Autodesk Inventor part; units mm, degrees
ref_plane "YZ Plane" through (0, 0, 0) normal (1, 0, 0) x (0, 1, 0)
ref_plane "XZ Plane" through (0, 0, 0) normal (0, 1, 0) x (-1, 0, 0)
ref_plane "XY Plane" through (0, 0, 0) normal (0, 0, 1) x (1, 0, 0)
sketch "Эскиз1" plane through (0, 0, 0) normal (1, 0, 0) x (0, 1, 0)
  line L0 (0.4, 16.4596) -> (0.4, 13.8596)
  line L1 (0.4, 13.8596) -> (2, 13.8596)
  line L2 (2, 13.8596) -> (2, 13.0596)
  line L3 (2, 13.0596) -> (5, 13.0596)
  line L4 (5, 13.0596) -> (5, 1)
  line L5 (5, 1) -> (2, 1)
  line L6 (2, 1) -> (2, 0)
  line L7 (2, 0) -> (0, 0)
  line L8 (0, 0) -> (0, 16.5)
  line L9 (0, -3.302) -> (0, 19.8121)
  arc A0 (0.4, 16.4596) -> (0, 16.5) centre (0, 14.5) ccw
  dimension "d0" = 16.5
  dimension "d1" = 0.8
  dimension "d2" = 2.6
  dimension "d3" = 0.8
  dimension "d4" = 10
  dimension "d5" = 4
  dimension "d6" = 1
  dimension "d7" = 4
  dimension "d13" = 2
revolve "Вращение1" add sketch "Эскиз1" angle 360 about axis through (0, 0, -10) along (0, 0, 1)
sketch "Эскиз2" plane through (0, 0, 1) normal (0, 0, -1) x (-1, 0, 0)
  circle A0 centre (0, 0) radius 5
  line L0 (-3, 4) -> (3, 4)
  line L1 (3, -4) -> (-3, -4)
  line L2 (7, 0) -> (-7, 0)
  dimension "d9" = 8
extrude "Выдавливание1" cut sketch "Эскиз2" against normal blind 13.25 contours L0 A0 | A0 L1
fillet "Сопряжение1" radius 0.5 12 edges at (0, 4, 13.0596) (5, 0, 13.0596) (-5, 0, 13.0596) (0, -4, 13.0596) (3, -4, 7.0298) (-3, -4, 7.0298) (-3, 4, 7.0298) (3, 4, 7.0298) (0, -4, 1) (5, 0, 1) (-5, 0, 1) (0, 4, 1)
properties part number "Моторчик" material "Латунь, мягкая, желтая"
For this review, take the finished solid that the model builds, in its own axes (mm). A direction names the side the tool comes from. Coordinates: 2 decimals unless noted, no trailing zeros. Write each loop counter-clockwise with the first axis right and the second up, starting at its lowest first coordinate (ties: lowest second). Pieces come first, ordered by that corner, then holes. Notation, with made-up numbers: (13.5, 67.5) -> (54.5, 67.5) arc R11 cw to (54.5, 82.5) -> close; hole circle Ø4 at (73.5, 61). An arc over 180 degrees is marked (long way). Write each question's results on one line, items separated by ' | '. Start each with the question number.
1) Consider section B-B (x = -1). Write out the cut boundary in (y, z), plus the area to 3 significant figures.
2) For faces 1 (the face through (-2, -1, 13.06)), 2 (the face through (0, 0, 0)), 3 (the face through (-2, -1, 1)), list the 3-axis set-ups (+Z, -Z, +X, -X, +Y, -Y) from which the entire face can be reached by the end or side of a thin tool; tool diameter is ignored.
3) Insertion check: pin 1 (2 mm diameter, centred on x = 3.5, z = 8, fed in from -Y). The pin has a flat end and moves straight along its axis. Give the tip position at first contact, or say it passes through.
4) The part is to be moulded in two halves that separate along Y. For faces 4 (the face through (0, 4, 7)), 5 (the face through (0.4, 0.4, 13.86)), 6 (the face through (0, -4, 7)), 7 (the face through (-1.952, -0.434, 0.493)), say which applies: +Y half, -Y half, draft (parallel to the pull), parting line (faces both ways), or undercut.
5) Wall thickness on L1, parallel to Z at x = 1.25, y = -2.5; L2, parallel to Z at x = -0.5, y = 0.75; L3, parallel to X at y = -1, z = 12: over which ranges is each line inside the solid? List them lowest first. Write a range as [from, to].
6) Consider section C-C (z = 15). Write out the cut boundary in (x, y), plus the area to 3 significant figures.
7) Consider section A-A (z = 10.5). Write out the cut boundary in (x, y), plus the area to 3 significant figures.
Geometry says:
1) outline: (-4, 1.5) arc R0.5 ccw to (-3.5, 1) -> (-1.73, 1) -> (-1.73, 0) -> (1.73, 0) -> (1.73, 1) -> (3.5, 1) arc R0.5 ccw to (4, 1.5) -> (4, 12.56) arc R0.5 ccw to (3.5, 13.06) -> (1.73, 13.06) -> (1.73, 13.86) -> (-1.73, 13.86) -> (-1.73, 13.06) -> (-3.5, 13.06) arc R0.5 ccw to (-4, 12.56) -> close | area: 102 mm^2
2) face 1: +Z | face 2: -Z, +X, -X, +Y, -Y | face 3: -Z
3) pin 1: y = -4
4) face 4: +Y half | face 5: draft | face 6: -Y half | face 7: parting line
5) L1: [1, 13.06] | L2: [0, 13.86] | L3: [-4.9, 4.9]
6) outline: circle Ø0.8 at (0, 0) | area: 0.503 mm^2
7) outline: (-3.14, -3.89) arc R0.5 ccw to (-2.83, -4) -> (2.83, -4) arc R0.5 ccw to (3.14, -3.89) arc R5 ccw to (3.14, 3.89) arc R0.5 ccw to (2.83, 4) -> (-2.83, 4) arc R0.5 ccw to (-3.14, 3.89) arc R5 ccw to start | area: 70.4 mm^2
